Input: part model. Units: mm. Frame: model coordinates. Face numbers are marked on the shaded views. A direction names the side the tool comes from. Give positions to 0.01 mm unless a question says otherwise; leave off trailing zeros. Write each loop counter-clockwise with the first axis right and the second up, starting at its lowest first coordinate (ties: lowest second). Pieces come first, ordered by that corner, then holes.
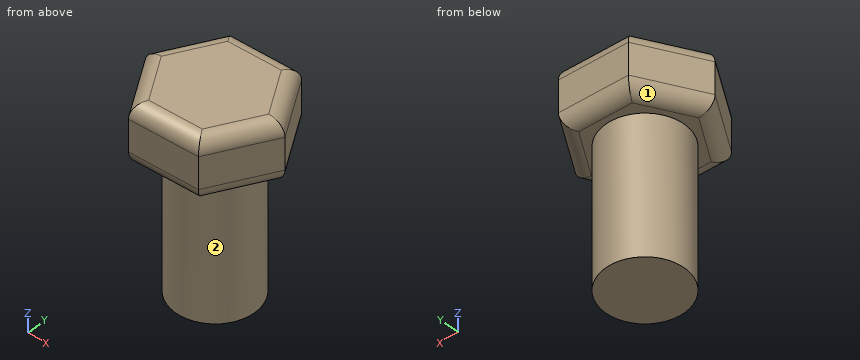
```python
from build123d import *

# Parameters (mm, degrees)
SKETCH1_R           = 2
BOSS_EXTRUDE1_DEPTH = 7
BOSS_EXTRUDE2_DEPTH = 3
FILLET1_R           = 0.7


with BuildPart() as part:
    # Sketch1 → Boss-Extrude1 (new body)
    with BuildSketch(Plane.XY):
        Circle(SKETCH1_R)
    extrude(amount=BOSS_EXTRUDE1_DEPTH)

    # Sketch2 → Boss-Extrude2 (add)
    with BuildSketch(Plane.XY.offset(7)):
        Polygon((-1.595912417, -3.074583477), (1.864711189, -2.919392434), (3.460623606, 0.155191044), (1.595912417, 3.074583477), (-1.864711189, 2.919392434), (-3.460623606, -0.155191044), align=None)
    extrude(amount=BOSS_EXTRUDE2_DEPTH)

    # Fillet1
    fillet1_edges = [part.edges().sort_by_distance(p)[0] for p in [
        (2.528268011, 1.614887261, 7),
        (-0.134399386, 2.996987955, 7),
        (-2.662667397, 1.382100695, 7),
        (-2.528268011, -1.614887261, 7),
        (0.134399386, -2.996987955, 7),
        (2.662667397, -1.382100695, 7),
        (2.528268011, 1.614887261, 10),
        (-0.134399386, 2.996987955, 10),
        (-2.662667397, 1.382100695, 10),
        (-2.528268011, -1.614887261, 10),
        (0.134399386, -2.996987955, 10),
        (2.662667397, -1.382100695, 10),
    ]]
    fillet(fillet1_edges, radius=FILLET1_R)


solid = part.part
```
Item 1: Section A-A (z = 7.5). Return loops of the section in (x, y), and give its area (3 significant figures).
Item 2: Section B-B (z = 6.25). Return loops of the section in (x, y).
Item 3: Ray query, line 1 (Z direction, x = 1.25, y = -1.75); line 2 (Y direction, x = 2, z = 9); line 3 (X direction, y = -1.5, z = 2.25). Return the intervals inside material, ascending.
Item 4: Set-up query: the marked faces 1 and 2. Return all of +Z, -Z, +X, -X, +Y, -Y with unobstructed straight access to the full face (end or side cutting, diameter ignored); none if empty.
Item 5: Pin query (flat end, axial travel): pin 1 (1.5 mm diameter, centred on x = 2, z = 3.5, fed in from -Y); pin 2 (1 mm diameter, centred on x = 2, z = 9, fed in from -Y); pin 3 (1.5 mm diameter, centred on y = -1, z = 4, fed in from -X). Return the tip coordinate at first contact, or that it passes through.
Solved:
1. outline: (-3.43, -0.15) - (-1.58, -3.04) - (1.85, -2.89) - (3.43, 0.15) - (1.58, 3.04) - (-1.85, 2.89) - close
1. area: 30.6 mm2
2. outline: circle Ø4 at (0, 0)
3. line 1: z = 7 to 10
3. line 2: y = -2.66 to 2.44
3. line 3: x = -1.32 to 1.32
4. face 1: -Z, -X, +Y
4. face 2: -Z
5. pin 1: stops at y = -1.56
5. pin 2: stops at y = -2.94
5. pin 3: stops at x = -1.98
